from build123d import *

# Parameters (mm, degrees)
BOSS_EXTRUDE1_DEPTH = 6.096
FILLET1_R           = 6.45
FILLET2_R           = 3.175


with BuildPart() as part:
    # Sketch1 → Boss-Extrude1 (new, symmetric)
    with BuildSketch(Plane.XY):
        Polygon((159.995567884, -85.917938074), (150.470567884, -69.420154132), (31.146005713, -138.312222222), (88.9, -138.312222222), (88.9, -150.504222222), (50.8, -150.504222222), (50.8, -163.204222222), (82.55, -163.204222222), (111.661584515, -328.304222222), (149.761584515, -328.304222222), (127, -104.967938074), align=None)
    extrude(amount=BOSS_EXTRUDE1_DEPTH, both=True)

    # Fillet1
    fillet1_edges = [part.edges().sort_by_distance(p)[0] for p in [
        (127, -104.967938074, 0),
        (31.146005713, -138.312222222, 0),
        (150.470567884, -69.420154132, 0),
        (159.995567884, -85.917938074, 0),
    ]]
    fillet(fillet1_edges, radius=FILLET1_R)

    # Fillet2
    fillet2_edges = [part.edges().sort_by_distance(p)[0] for p in [
        (82.55, -163.204222222, 0),
        (50.8, -163.204222222, 0),
    ]]
    fillet(fillet2_edges, radius=FILLET2_R)


solid = part.part
Input: part model. Units: mm. Frame: model coordinates. A direction names the side the tool comes from. Give positions to 0.01 mm unless a question says otherwise; leave off trailing zeros. Write each loop counter-clockwise with the first axis right and the second up, starting at its lowest first coordinate (ties: lowest second). Pieces come first, ordered by that corner, then holes. Notation, with made-up numbers: M 22.25,58 L 69.25,58 A14 cw 69.25,85 Z; hole C -30.5,-25 d2. An arc over 180 degrees is marked long. Write item = value, one per line. Start each with the question number.
1) Material intervals for line 1 along Y through (x, z) = (78, -3.25); line 2 along Y through (x, z) = (77.5, -3.75); line 3 along X through (y, z) = (-153, 4), sorted ascending. Write a range as [from, to].
2) First-contact query: pin 1 Ø2 at (y, z) = (-102.5, -0.5) entering from +X; pin 2 Ø1.5 at (y, z) = (-150.5, -3.5) entering from +X; pin 3 Ø3 at (x, z) = (74.5, -1) entering from +Y. Flat tips, straight axial feed; report the tip coordinate or a pass-through.
3) Cut plane C-C on x = 58.5. Return the cut outline in (y, z), then the cut area to 3 significant figures.
4) Draft query along Y for faces 1 (the cylindrical face through (157.433, -85.158, -0.085)), 2 (the flat face through (155.255, -77.706, 0.085)), 3 (the flat face through (88.9, -144, 0)). Return one class per face: +Y half, -Y half, draft (parallel to the pull), parting line (faces both ways), or undercut.
5) Cut plane B-B on z = -4.25. Return the cut outline in (x, y) (3 decimals).
6) Reachability of faces 4 (the flat face through (142.346, -96.108, 0.085)), 5 (the flat face through (72, -138.312, 0)), 6 (the flat face through (67, -163.204, 0)) from +Z, -Z, +X, -X, +Y, -Y: full face, straight path, thin tool, end or side. Return the list, or none.
7) Cut plane A-A on x = 139.5. Return the cut outline in (y, z).
8) Cut plane D-D on y = -282. Return the cut outline in (x, z).
Solved:
q1.line_1 = [-163.2, -150.5], [-138.31, -111.26]
q1.line_2 = [-163.2, -150.5], [-138.31, -111.55]
q1.line_3 = [50.8, 131.9]
q2.pin_1 = 133.01
q2.pin_2 = 131.72
q2.pin_3 = -112.42
q3.outline = M -163.2,-6.1 L -150.5,-6.1 L -150.5,6.1 L -163.2,6.1 Z; M -138.31,-6.1 L -122.52,-6.1 L -122.52,6.1 L -138.31,6.1 Z
q3.area = 347 mm2
q4.face_1 = parting line
q4.face_2 = +Y half
q4.face_3 = undercut
q5.outline = M 50.8,-160.029 A3.175 ccw 53.975,-163.204 L 79.886,-163.204 A3.175 cw 83.013,-165.828 L 111.662,-328.304 L 149.762,-328.304 L 127.423,-109.121 A6.45 cw 130.615,-102.881 L 154.41,-89.143 A6.45 ccw 156.771,-80.332 L 153.696,-75.006 A6.45 ccw 144.885,-72.645 L 51.993,-126.276 A6.45 ccw 55.218,-138.312 L 88.9,-138.312 L 88.9,-150.504 L 50.8,-150.504 Z
q6.face_4 = +Z, -Z, +X
q6.face_5 = +Z, -Z, -X
q6.face_6 = +Z, -Z, -X, -Y
q7.outline = M -328.3,-6.1 L -227.62,-6.1 L -227.62,6.1 L -328.3,6.1 Z; M -97.75,-6.1 L -75.75,-6.1 L -75.75,6.1 L -97.75,6.1 Z
q8.outline = M 103.5,-6.1 L 145.04,-6.1 L 145.04,6.1 L 103.5,6.1 Z
